CAD build for the part. Positions are in the model's coordinates, mm. Face numbers are marked on the shaded views. A direction names the side the tool comes from. Give positions to 0.01 mm unless a question says otherwise; leave off trailing zeros. Order: outer loops, then holes, each group sorted by start corner. A loop starts at its lowest first (then second) coordinate and runs counter-clockwise, first axis right, second up.
Item 1: Band-saw the part on A-A on z = -35. Give the cut face in (x, y).
Item 2: Band-saw the part on C-C on y = 15. Give the cut face in (x, z).
Item 3: Band-saw the part on B-B on y = 7.5. Give the cut face in (x, z).
Item 4: Flat gauge pins, fed straight in: P1, Ø8, axis at y = 9, z = -24, coming from the -X side; P2, Ø12, axis at y = 13.5, z = -20, coming from the +X side; P3, Ø6, axis at y = 28.5, z = -28.5, coming from the -X side. Where does each tip first touch, or does it go through?
Item 5: Which spindle directions (+Z, -Z, +X, -X, +Y, -Y) get a long thin tool onto all of the face, cutting with end or side? Do the marked faces 1, 2 and 3. Say none if no direction does.
Item 6: Band-saw the part on D-D on x = -30.5. Give the cut face in (y, z).
Item 7: Two-plate mould, pull along Z, no slides. Class the marked faces 4, 5 and 6: released by +Z, released by -Z, zero draft, split by the parting line, or undercut.
Item 8: Wall check: L1, parallel to X at y = 26, z = -10; L2, parallel to X at y = 17, z = -14.5; L3, parallel to Y at x = 2, z = -19. Give the ranges that are in metal, low to high.
```python
from build123d import *

# Parameters (mm, degrees)
SKETCH3_W           = 100
SKETCH3_H           = 40
SKETCH3_R           = 3
BOSS_EXTRUDE1_DEPTH = 5
FLEX1_START         = -36
FLEX1_OUTLINE_W     = 48.866197724
FLEX1_OUTLINE_H     = 40
FLEX1_DEPTH         = 33.40315081
FLEX1_START_2       = -2.59684919
FLEX1_2_OUTLINE_W   = 48.866197724
FLEX1_2_OUTLINE_H   = 40
FLEX1_2_OUTLINE_R   = 3
FLEX1_2_DEPTH       = 8.866197724
FLEX1_START_3       = 2.448182419
FLEX1_3_OUTLINE_W   = 5
FLEX1_3_OUTLINE_H   = 40
FLEX1_3_DEPTH       = 48.821166115
FLEX1_START_4       = -51.269348534
FLEX1_4_OUTLINE_W   = 3.866197724
FLEX1_4_OUTLINE_H   = 40
FLEX1_4_DEPTH       = 45
FLEX1_START_5       = 2.59684919
FLEX1_5_OUTLINE_R   = 3
FLEX1_5_OUTLINE_W   = 3.821166115
FLEX1_5_OUTLINE_H   = 40
FLEX1_5_DEPTH       = 33.40315081
FLEX1_START_6       = -2.40315081
FLEX1_6_OUTLINE_R   = 3
FLEX1_6_DEPTH       = 5
FLEX1_START_7       = 1.935784603
FLEX1_7_OUTLINE_W   = 0.045031609
FLEX1_7_OUTLINE_H   = 40
FLEX1_7_DEPTH       = 0.545856358
FLEX1_START_8       = -40
FLEX1_8_DEPTH       = 40
BOSS_EXTRUDE2_DEPTH = 1.5


with BuildPart() as part:
    # Sketch3 → Boss-Extrude1 (new body)
    with BuildSketch(Plane(origin=(0, 0, 0), x_dir=(1, 0, 0), z_dir=(0, 1, 0))):
        with Locations((0, 20)):
            Rectangle(SKETCH3_W, SKETCH3_H)
        with Locations(Location((35, 30, 0), (0, 0, 270))):
            Circle(SKETCH3_R, mode=Mode.SUBTRACT)
        with Locations(Location((35, 10.435948304, 0), (0, 0, 270))):
            Circle(SKETCH3_R, mode=Mode.SUBTRACT)
        with Locations(Location((-35, 10.435948304, 0), (0, 0, 90))):
            Circle(SKETCH3_R, mode=Mode.SUBTRACT)
        with Locations(Location((-35, 30, 0), (0, 0, 90))):
            Circle(SKETCH3_R, mode=Mode.SUBTRACT)
    extrude(amount=BOSS_EXTRUDE1_DEPTH)

    # Flex1: read off the stored shape, not the designer's step
    # Flex1 outline → Flex1 (cut)
    with BuildSketch(Plane(origin=(0, 0, 0), x_dir=(0.707106781186546, -0.707106781186549, 0), z_dir=(0.707106781186549, 0.707106781186546, 0)).offset(FLEX1_START)):
        with Locations((-26.836249672, 20)):
            Rectangle(FLEX1_OUTLINE_W, FLEX1_OUTLINE_H)
    extrude(amount=FLEX1_DEPTH, mode=Mode.SUBTRACT)

    # Flex1 2 outline → Flex1 2 (add)
    with BuildSketch(Plane(origin=(0, 0, 0), x_dir=(0.707106781186546, -0.707106781186549, 0), z_dir=(0.707106781186549, 0.707106781186546, 0)).offset(FLEX1_START_2)):
        with Locations((-26.836249672, 20)):
            Rectangle(FLEX1_2_OUTLINE_W, FLEX1_2_OUTLINE_H)
        with Locations((-36.269348534, 10.435948304)):
            Circle(FLEX1_2_OUTLINE_R, mode=Mode.SUBTRACT)
        with Locations((-36.269348534, 30)):
            Circle(FLEX1_2_OUTLINE_R, mode=Mode.SUBTRACT)
    extrude(amount=FLEX1_2_DEPTH)

    # Flex1 3 outline → Flex1 3 (add)
    with BuildSketch(Plane(origin=(0, 0, 0), x_dir=(0.707106781186546, -0.707106781186549, 0), z_dir=(0.707106781186549, 0.707106781186546, 0)).offset(FLEX1_START_3)):
        with Locations((0.09684919, 20)):
            Rectangle(FLEX1_3_OUTLINE_W, FLEX1_3_OUTLINE_H)
    extrude(amount=FLEX1_3_DEPTH)

    # Flex1 4 outline → Flex1 4 (cut)
    with BuildSketch(Plane(origin=(0, 0, 0), x_dir=(0.707106781186546, 0.707106781186549, 0), z_dir=(0.707106781186549, -0.707106781186546, 0)).offset(FLEX1_START_4)):
        with Locations((4.336249672, -20)):
            Rectangle(FLEX1_4_OUTLINE_W, FLEX1_4_OUTLINE_H)
    extrude(amount=FLEX1_4_DEPTH, mode=Mode.SUBTRACT)

    # Flex1 5 outline → Flex1 5 (cut)
    with BuildSketch(Plane(origin=(0, 0, 0), x_dir=(0.707106781186546, 0.707106781186549, 0), z_dir=(0.707106781186549, -0.707106781186546, 0)).offset(FLEX1_START_5)):
        with Locations((36.269348534, -10.435948304)):
            Circle(FLEX1_5_OUTLINE_R)
        with Locations((36.269348534, -30)):
            Circle(FLEX1_5_OUTLINE_R)
        with Locations((4.358765477, -20)):
            Rectangle(FLEX1_5_OUTLINE_W, FLEX1_5_OUTLINE_H)
    extrude(amount=FLEX1_5_DEPTH, mode=Mode.SUBTRACT)

    # Flex1 6 outline → Flex1 6 (cut)
    with BuildSketch(Plane(origin=(0, 0, 0), x_dir=(0.707106781186546, 0.707106781186549, 0), z_dir=(0.707106781186549, -0.707106781186546, 0)).offset(FLEX1_START_6)):
        with Locations((36.269348534, -10.435948304)):
            Circle(FLEX1_6_OUTLINE_R)
        with Locations((36.269348534, -30)):
            Circle(FLEX1_6_OUTLINE_R)
    extrude(amount=FLEX1_6_DEPTH, mode=Mode.SUBTRACT)

    # Flex1 7 outline → Flex1 7 (cut)
    with BuildSketch(Plane(origin=(0, 0, 0), x_dir=(0.707106781186546, 0.707106781186549, 0), z_dir=(0.707106781186549, -0.707106781186546, 0)).offset(FLEX1_START_7)):
        with Locations((2.425666614, -20)):
            Rectangle(FLEX1_7_OUTLINE_W, FLEX1_7_OUTLINE_H)
    extrude(amount=FLEX1_7_DEPTH, mode=Mode.SUBTRACT)

    # Flex1 8 outline → Flex1 8 (cut)
    with BuildSketch(Plane.XY.offset(FLEX1_START_8)):
        with BuildLine():
            ThreePointArc((-2.733814628, 6.132383096), (0, 5), (2.733814628, 6.132383096))
            Line((2.733814628, 6.132383096), (0, 8.866197724))
            Line((0, 8.866197724), (-2.733814628, 6.132383096))
        make_face()
        with BuildLine():
            Line((3.567376062, -0.105123282), (6.269348534, 2.59684919))
            ThreePointArc((6.269348534, 2.59684919), (3.392946977, 0.674899116), (0, 0))
            Line((0, 0), (3.398568468, 0))
            Line((3.398568468, 0), (3.068090654, 0.330477814))
            Line((3.068090654, 0.330477814), (3.09993281, 0.36231997))
            Line((3.09993281, 0.36231997), (3.567376062, -0.105123282))
        make_face()
        with BuildLine():
            Line((-3.398568468, 0), (0, 0))
            ThreePointArc((0, 0), (-3.392946977, 0.674899116), (-6.269348534, 2.59684919))
            Line((-6.269348534, 2.59684919), (-3.535533906, -0.136965438))
            Line((-3.535533906, -0.136965438), (-3.398568468, 0))
        make_face()
        Polygon((8.672499344, 5), (6.269348534, 2.59684919), (8.866197724, 0), (50, 0), (50, 5), align=None)
    extrude(amount=FLEX1_8_DEPTH, mode=Mode.SUBTRACT)

    # Sketch4 → Boss-Extrude2 (add, symmetric)
    with BuildSketch(Plane.XY.offset(-10)):
        Polygon((0, 0), (10.606601718, 10.606601718), (-10.606601718, 10.606601718), align=None)
    boss_extrude2 = extrude(amount=BOSS_EXTRUDE2_DEPTH, both=True)

    # Mirror1: Boss-Extrude2 across plane
    add(boss_extrude2.mirror(Plane.XY.offset(-20)))


solid = part.part
```
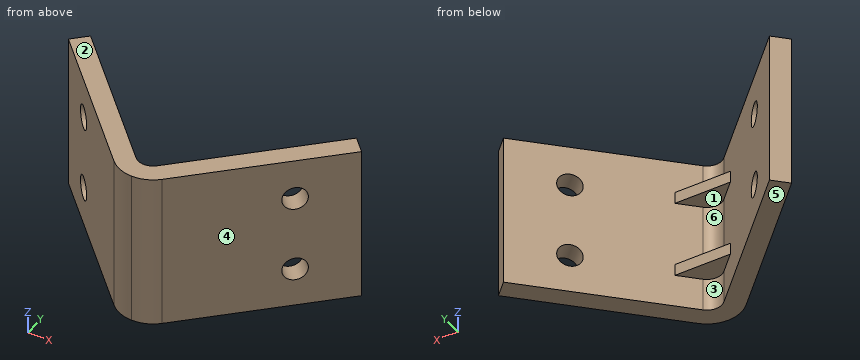
The answers:
1. outline: (-38.09, 34.42) - (-6.27, 2.6) arc R8.87 ccw to (6.27, 2.6) - (38.09, 34.42) - (34.55, 37.95) - (2.73, 6.13) arc R3.87 cw to (-2.73, 6.13) - (-34.55, 37.95) - close
2. outline: (-18.67, -40) - (-11.6, -40) - (-11.6, 0) - (-18.67, 0) - close; (11.6, -40) - (18.67, -40) - (18.67, 0) - (11.6, 0) - close
3. outline: (-11.17, -40) - (-4.1, -40) - (-4.1, -31.5) - (4.1, -31.5) - (4.1, -40) - (11.17, -40) - (11.17, 0) - (4.1, 0) - (4.1, -8.5) - (-4.1, -8.5) - (-4.1, 0) - (-11.17, 0) - close; hole (-4.1, -28.5) - (4.1, -28.5) - (4.1, -11.5) - (-4.1, -11.5) - close
4. P1: stops at x = -16.67
4. P2: stops at x = 23.17
4. P3: stops at x = -35.17
5. face 1: +Y
5. face 2: +Z, +X, -X, +Y, -Y
5. face 3: -Z, +Y
6. outline: (26.83, -40) - (33.9, -40) - (33.9, 0) - (26.83, 0) - close
7. face 4: zero draft
7. face 5: released by -Z
7. face 6: undercut
8. L1: x = -29.67 to -29.49, 29.49 to 29.67
8. L2: x = -20.67 to -13.6, 13.6 to 20.67
8. L3: y = 0.23 to 5.56
